```python
from build123d import *

# Parameters (mm, degrees)
ESQUISSE1_R        = 10.5
ESQUISSE1_R_2      = 3.4
ESQUISSE1_R_3      = 1.925
BOSS_EXTRU_2_DEPTH = 5


with BuildPart() as part:
    # Esquisse1 → Boss.-Extru.2 (new body)
    with BuildSketch(Plane.XY):
        with BuildLine():
            Line((50, -44.919487431), (50, -33.862050579))
            ThreePointArc((50, -33.862050579), (49.777389032, -32.945051), (49.159111773, -32.232185585))
            ThreePointArc((49.159111773, -32.232185585), (45.31641316, -26.748192273), (45.795558863, -20.069050512))
            ThreePointArc((45.795558863, -20.069050512), (48.937602838, -10.252366967), (50, 0))
            ThreePointArc((50, 0), (48.936869799, 10.255865358), (45.79268903, 20.075597908))
            ThreePointArc((45.79268903, 20.075597908), (45.313248124, 26.757056992), (49.158537806, 32.242082639))
            ThreePointArc((49.158537806, 32.242082639), (49.777227562, 32.955043184), (50, 33.872355669))
            Line((50, 33.872355669), (50, 44.919487431))
            ThreePointArc((50, 44.919487431), (48.51195232, 48.51195232), (44.919487431, 50))
            Line((44.919487431, 50), (33.862050579, 50))
            ThreePointArc((33.862050579, 50), (32.945051, 49.777389032), (32.232185585, 49.159111773))
            ThreePointArc((32.232185585, 49.159111773), (26.748192273, 45.31641316), (20.069050512, 45.795558863))
            ThreePointArc((20.069050512, 45.795558863), (10.252366967, 48.937602838), (0, 50))
            ThreePointArc((0, 50), (-10.255865358, 48.936869799), (-20.075597908, 45.79268903))
            ThreePointArc((-20.075597908, 45.79268903), (-26.757056992, 45.313248124), (-32.242082639, 49.158537806))
            ThreePointArc((-32.242082639, 49.158537806), (-32.955043184, 49.777227562), (-33.872355669, 50))
            Line((-33.872355669, 50), (-44.919487431, 50))
            ThreePointArc((-44.919487431, 50), (-48.51195232, 48.51195232), (-50, 44.919487431))
            Line((-50, 44.919487431), (-50, 33.862050579))
            ThreePointArc((-50, 33.862050579), (-49.777389032, 32.945051), (-49.159111773, 32.232185585))
            ThreePointArc((-49.159111773, 32.232185585), (-45.31641316, 26.748192273), (-45.795558863, 20.069050512))
            ThreePointArc((-45.795558863, 20.069050512), (-48.937602838, 10.252366967), (-50, 0))
            ThreePointArc((-50, 0), (-48.936869799, -10.255865358), (-45.79268903, -20.075597908))
            ThreePointArc((-45.79268903, -20.075597908), (-45.313248124, -26.757056992), (-49.158537806, -32.242082639))
            ThreePointArc((-49.158537806, -32.242082639), (-49.777227562, -32.955043184), (-50, -33.872355669))
            Line((-50, -33.872355669), (-50, -44.919487431))
            ThreePointArc((-50, -44.919487431), (-48.51195232, -48.51195232), (-44.919487431, -50))
            Line((-44.919487431, -50), (-33.862050579, -50))
            ThreePointArc((-33.862050579, -50), (-32.945051, -49.777389032), (-32.232185585, -49.159111773))
            ThreePointArc((-32.232185585, -49.159111773), (-26.748192273, -45.31641316), (-20.069050512, -45.795558863))
            ThreePointArc((-20.069050512, -45.795558863), (-10.252366967, -48.937602838), (0, -50))
            ThreePointArc((0, -50), (10.255865358, -48.936869799), (20.075597908, -45.79268903))
            ThreePointArc((20.075597908, -45.79268903), (26.757056992, -45.313248124), (32.242082639, -49.158537806))
            ThreePointArc((32.242082639, -49.158537806), (32.955043184, -49.777227562), (33.872355669, -50))
            Line((33.872355669, -50), (44.919487431, -50))
            ThreePointArc((44.919487431, -50), (48.51195232, -48.51195232), (50, -44.919487431))
        make_face()
        Circle(ESQUISSE1_R, mode=Mode.SUBTRACT)
        with Locations((40, -40)):
            Circle(ESQUISSE1_R_2, mode=Mode.SUBTRACT)
        with Locations((-40, -40)):
            Circle(ESQUISSE1_R_2, mode=Mode.SUBTRACT)
        with Locations((0, 14.5)):
            Circle(ESQUISSE1_R_3, mode=Mode.SUBTRACT)
        with Locations((40, 40)):
            Circle(ESQUISSE1_R_2, mode=Mode.SUBTRACT)
        with Locations((-40, 40)):
            Circle(ESQUISSE1_R_2, mode=Mode.SUBTRACT)
        with Locations((12.557368355, -7.25)):
            Circle(ESQUISSE1_R_3, mode=Mode.SUBTRACT)
        with Locations((-12.557368355, -7.25)):
            Circle(ESQUISSE1_R_3, mode=Mode.SUBTRACT)
        with BuildLine():
            Line((29.746951244, -33.28248515), (19.14034941, -22.675883316))
            ThreePointArc((19.14034941, -22.675883316), (19.14034941, -19.14034941), (22.675883316, -19.14034941))
            Line((22.675883316, -19.14034941), (33.282485034, -29.746951128))
            ThreePointArc((33.282485034, -29.746951128), (33.282485209, -33.282485092), (29.746951244, -33.28248515))
        make_face(mode=Mode.SUBTRACT)
        with BuildLine():
            Line((-33.28248515, -29.746951244), (-22.675883316, -19.14034941))
            ThreePointArc((-22.675883316, -19.14034941), (-19.14034941, -19.14034941), (-19.14034941, -22.675883316))
            Line((-19.14034941, -22.675883316), (-29.746951128, -33.282485034))
            ThreePointArc((-29.746951128, -33.282485034), (-33.282485092, -33.282485209), (-33.28248515, -29.746951244))
        make_face(mode=Mode.SUBTRACT)
        with BuildLine():
            Line((33.28248515, 29.746951244), (22.675883316, 19.14034941))
            ThreePointArc((22.675883316, 19.14034941), (19.14034941, 19.14034941), (19.14034941, 22.675883316))
            Line((19.14034941, 22.675883316), (29.746951128, 33.282485034))
            ThreePointArc((29.746951128, 33.282485034), (33.282485092, 33.282485209), (33.28248515, 29.746951244))
        make_face(mode=Mode.SUBTRACT)
        with BuildLine():
            Line((-29.746951244, 33.28248515), (-19.14034941, 22.675883316))
            ThreePointArc((-19.14034941, 22.675883316), (-19.14034941, 19.14034941), (-22.675883316, 19.14034941))
            Line((-22.675883316, 19.14034941), (-33.282485034, 29.746951128))
            ThreePointArc((-33.282485034, 29.746951128), (-33.282485209, 33.282485092), (-29.746951244, 33.28248515))
        make_face(mode=Mode.SUBTRACT)
    extrude(amount=BOSS_EXTRU_2_DEPTH)


solid = part.part
```
CAD build for the part. Positions are in the model's coordinates, mm. A direction names the side the tool comes from. Round coordinates to 2 decimals unless told otherwise and drop trailing zeros. Order: outer loops, then holes, each group sorted by start corner. A loop starts at its lowest first (then second) coordinate and runs counter-clockwise, first axis right, second up.
Q1. Slice it at C-C (y = 8). Write the cut outline in (x, z).
Q2. Wall check: L1, parallel to Y at x = 40, z = 1.25; L2, parallel to Y at x = -42, z = 4.85; L3, parallel to Y at x = 12, z = 4.7. Give the ranges that are in metal, low to high.
Q3. Drop flat-ended pins along their axis: pin 1 (2.5 mm diameter, centred on x = 12.56, y = -7.25, fed in from +Z); pin 2 (1.5 mm diameter, centred on y = -9.5, z = 1.5, fed in from +X). Give the stop position or say it passes through.
Q4. Two-plate mould, pull along Y, no slides. Class faces 1 (the flat face through (50, 39, 2)), 2 (the cylindrical face through (-48.472, 48.551, 2.465)), 3 (the flat face through (24.518, -28.053, 2.465)): pulls with the +Y half, pulls with the -Y half, needs draft (parallel to the pull), parting line crosses it, or undercut.
Q5. Slice it at D-D (x = -4). Write the cut outline in (y, z).
Q6. Slice it at A-A (x = 40). Write the cut outline in (y, z).
Q7. Which spindle directions (+Z, -Z, +X, -X, +Y, -Y) get a long thin tool onto all of the face, cutting with end or side? Do faces 4 (the flat face through (-27.905, 24.369, 2.465)), 5 (the flat face through (-50, -39, 2)). Say none if no direction does.
Results below:
1. outline: (-49.36, 0) - (-6.8, 0) - (-6.8, 5) - (-49.36, 5) - close; (6.8, 0) - (49.36, 0) - (49.36, 5) - (6.8, 5) - close
2. L1: y = -50 to -43.4, -36.6 to 36.6, 43.4 to 50
2. L2: y = -50 to -42.75, -37.25 to 37.25, 42.75 to 50
2. L3: y = -48.54 to -9.09, -5.41 to 48.54
3. pin 1: passes through
3. pin 2: stops at x = 49.23
4. face 1: needs draft
4. face 2: pulls with the +Y half
4. face 3: undercut
5. outline: (-49.84, 0) - (-9.71, 0) - (-9.71, 5) - (-49.84, 5) - close; (9.71, 0) - (49.84, 0) - (49.84, 5) - (9.71, 5) - close
6. outline: (-50, 0) - (-43.4, 0) - (-43.4, 5) - (-50, 5) - close; (-36.6, 0) - (36.6, 0) - (36.6, 5) - (-36.6, 5) - close; (43.4, 0) - (50, 0) - (50, 5) - (43.4, 5) - close
7. face 4: +Z, -Z
7. face 5: +Z, -Z, -X, +Y, -Y
